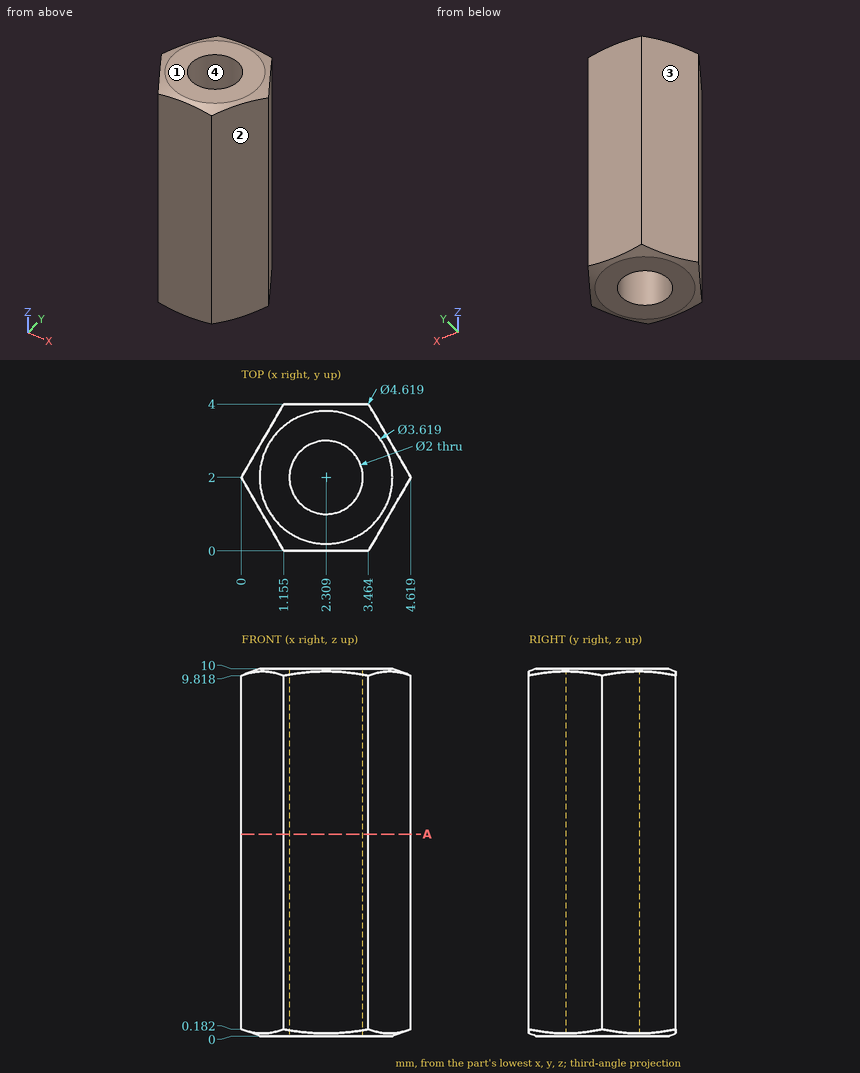
For this review, use the dimensioned drawing (mm, ordinates from the lowest corner) and the shaded views. Give positions to 0.01 mm unless a question says otherwise; leave off trailing zeros. Write each loop counter-clockwise with the first axis right and the second up, starting at its lowest first coordinate (ties: lowest second). Pieces come first, ordered by that corner, then holes. Notation, with made-up numbers: M -24.5,44 L 32.5,44 A20 cw 32.5,52 Z; hole C 89,-15 d4. An arc over 180 degrees is marked long. Write item = value, one per line. Start each with the question number.
Q1. Clearance check with a flat-ended pin moving along its axis: pin 1 (1.2 mm diameter, centred on x = 2.31, y = 2, fed in from +Z). State where the tip first meets the part, or that it passes through.
Q2. Mouldability with a two-part tool opening along X and no side actions: class the marked faces 1, 2, 3 and 4 as released by +X, released by -X, zero draft, split by the parting line, or undercut.
Q3. For line 1 (Y direction, x = 1.85, z = 2); line 2 (X direction, y = 2.45, z = 7) (1 decimal); line 3 (X direction, y = 2.1, z = 4) (1 decimal), list the stretches that pass through material, from the lowest coordinate up.
Q4. We need section A-A (z = 5.5). State the section outline as (x, y) points (1 decimal).
Result set:
q1.pin_1 = through
q2.face_1 = zero draft
q2.face_2 = released by +X
q2.face_3 = released by -X
q2.face_4 = undercut
q3.line_1 = 0 to 1.11, 2.89 to 4
q3.line_2 = 0.3 to 1.4, 3.2 to 4.4
q3.line_3 = 0.1 to 1.3, 3.3 to 4.6
q4.outline = M 0,2 L 1.2,0 L 3.5,0 L 4.6,2 L 3.5,4 L 1.2,4 Z; hole C 2.3,2 d2
